Work out the finished part from the listing and answer in its coordinate system (mm). A direction names the side the tool comes from. Round coordinates to 2 decimals unless told otherwise and drop trailing zeros. Loops run counter-clockwise (first coordinate to the right, second up) from the corner with the lowest first, then second, coordinate; pieces in that order, holes last. Notation, with made-up numbers: (0, 10) - (27, 10) arc R19 ccw to (27, 42) - close; hole circle Ø10 at (21, 9.5). An arc over 180 degrees is marked (long way). Return JSON: item names as keys, results as strings.
from build123d import *

# Parameters (mm, degrees)
BOSS_EXTRUDE1_DEPTH      = 5
BOSS_EXTRUDE1_DEPTH_BACK = 5
SKETCH1_W                = 32.8
SKETCH1_H                = 137
CUT_EXTRUDE1_DEPTH       = 2.8
CUT_EXTRUDE1_DEPTH_BACK  = 2.8
SKETCH1_4_R              = 4.9
CUT_EXTRUDE3_DEPTH       = 2.8
CUT_EXTRUDE3_DEPTH_BACK  = 2.8
SKETCH1_8_W              = 2
SKETCH1_8_H              = 2
SKETCH1_8_W_2            = 9.8
BOSS_EXTRUDE2_START      = 2.6
SKETCH1_5_W              = 8.1
SKETCH1_5_H              = 8.6
SKETCH1_5_R              = 2.15
BOSS_EXTRUDE2_DEPTH      = 2.4
BOSS_EXTRUDE3_START      = -5
SKETCH1_6_W              = 8.1
SKETCH1_6_H              = 8.6
SKETCH1_6_R              = 2.15
BOSS_EXTRUDE3_DEPTH      = 2.4
FILLET1_R                = 5
CUT_EXTRUDE4_DEPTH       = 141.960419977
CUT_EXTRUDE4_DEPTH_BACK  = 141.960419977
SKETCH3_R                = 2.15


with BuildPart() as part:
    # Sketch1 → Boss-Extrude1 (new, two sides: drawn at the far end of the back side and taken through both)
    with BuildSketch(Plane(origin=(0, 0, 0), x_dir=(1, 0, 0), z_dir=(0, 1, 0)).offset(-BOSS_EXTRUDE1_DEPTH_BACK)):
        with Locations((16.4, -68.5)):
            Rectangle(SKETCH1_W, SKETCH1_H)
        with BuildLine():
            Line((9, -135), (9, -10.5))
            ThreePointArc((9, -10.5), (13.9, -5.6), (18.8, -10.5))
            Line((18.8, -10.5), (18.8, -135))
            Line((18.8, -135), (9, -135))
        make_face(mode=Mode.SUBTRACT)
    extrude(amount=BOSS_EXTRUDE1_DEPTH + BOSS_EXTRUDE1_DEPTH_BACK)

    # Sketch1<4> → Cut-Extrude1 (cut, two sides: drawn at the far end of the back side and taken through both)
    with BuildSketch(Plane(origin=(0, 0, 0), x_dir=(1, 0, 0), z_dir=(0, 1, 0)).offset(-CUT_EXTRUDE1_DEPTH_BACK)):
        with BuildLine():
            Line((7, -10.5), (7, -135))
            Line((7, -135), (9, -135))
            Line((9, -135), (9, -15.357983121))
            ThreePointArc((9, -15.357983121), (7.519561144, -13.126785107), (7, -10.5))
        make_face()
        with BuildLine():
            Line((18.8, -135), (20.8, -135))
            Line((20.8, -135), (20.8, -10.5))
            ThreePointArc((20.8, -10.5), (20.280438856, -13.126785107), (18.8, -15.357983121))
            Line((18.8, -15.357983121), (18.8, -135))
        make_face()
        with BuildLine():
            Line((9, -15.357983121), (9, -135))
            Line((9, -135), (18.8, -135))
            Line((18.8, -135), (18.8, -15.357983121))
            ThreePointArc((18.8, -15.357983121), (13.9, -17.4), (9, -15.357983121))
        make_face()
        with BuildLine():
            ThreePointArc((20.8, -10.5), (13.9, -3.6), (7, -10.5))
            ThreePointArc((7, -10.5), (7.519561144, -13.126785107), (9, -15.357983121))
            Line((9, -15.357983121), (9, -10.5))
            ThreePointArc((9, -10.5), (13.9, -5.6), (18.8, -10.5))
            Line((18.8, -10.5), (18.8, -15.357983121))
            ThreePointArc((18.8, -15.357983121), (20.280438856, -13.126785107), (20.8, -10.5))
        make_face()
        with BuildLine():
            Line((9, -10.5), (9, -15.357983121))
            ThreePointArc((9, -15.357983121), (13.9, -17.4), (18.8, -15.357983121))
            Line((18.8, -15.357983121), (18.8, -10.5))
            ThreePointArc((18.8, -10.5), (13.9, -15.4), (9, -10.5))
        make_face()
        with Locations((13.9, -10.5)):
            Circle(SKETCH1_4_R)
    extrude(amount=CUT_EXTRUDE1_DEPTH + CUT_EXTRUDE1_DEPTH_BACK, mode=Mode.SUBTRACT)

    # Sketch1<8> → Cut-Extrude3 (cut, two sides: drawn at the far end of the back side and taken through both)
    with BuildSketch(Plane(origin=(0, 0, 0), x_dir=(1, 0, 0), z_dir=(0, 1, 0)).offset(-CUT_EXTRUDE3_DEPTH_BACK)):
        with Locations((8, -136)):
            Rectangle(SKETCH1_8_W, SKETCH1_8_H)
        with Locations((19.8, -136)):
            Rectangle(SKETCH1_8_W, SKETCH1_8_H)
        with Locations((13.9, -136)):
            Rectangle(SKETCH1_8_W_2, SKETCH1_8_H)
    extrude(amount=CUT_EXTRUDE3_DEPTH + CUT_EXTRUDE3_DEPTH_BACK, mode=Mode.SUBTRACT)

    # Sketch1<5> → Boss-Extrude2 (add)
    with BuildSketch(Plane(origin=(0, 0, 0), x_dir=(1, 0, 0), z_dir=(0, 1, 0)).offset(BOSS_EXTRUDE2_START)):
        with Locations((20.25, 4.3)):
            Rectangle(SKETCH1_5_W, SKETCH1_5_H)
        with Locations(Location((20.25, 4.55, 0), (0, 0, 270))):
            Circle(SKETCH1_5_R, mode=Mode.SUBTRACT)
    extrude(amount=BOSS_EXTRUDE2_DEPTH)

    # Sketch1<6> → Boss-Extrude3 (add)
    with BuildSketch(Plane(origin=(0, 0, 0), x_dir=(1, 0, 0), z_dir=(0, 1, 0)).offset(BOSS_EXTRUDE3_START)):
        with Locations((20.25, 4.3)):
            Rectangle(SKETCH1_6_W, SKETCH1_6_H)
        with Locations(Location((20.25, 4.55, 0), (0, 0, 270))):
            Circle(SKETCH1_6_R, mode=Mode.SUBTRACT)
    extrude(amount=BOSS_EXTRUDE3_DEPTH)

    # Mirror1: part across plane


with BuildPart() as part_1:
    add(part.part)
    add(part.part.mirror(Plane(origin=(0, 0, 0), x_dir=(0, 0, 1), z_dir=(1, 0, 0))))

    # Fillet1
    fillet1_edges = [part_1.edges().sort_by_distance(p)[0] for p in [
        (-7, 0, 137),
        (7, 0, 137),
    ]]
    fillet(fillet1_edges, radius=FILLET1_R)

    # Sketch3 → Cut-Extrude4 (cut, two sides: drawn at the far end of the back side and taken through both)
    with BuildSketch(Plane(origin=(0, 0, 0), x_dir=(1, 0, 0), z_dir=(0, 1, 0)).offset(-CUT_EXTRUDE4_DEPTH_BACK)):
        with Locations(Location((0, -132, 0), (0, 0, 270))):
            Circle(SKETCH3_R)
        with Locations(Location((26.8, -132, 0), (0, 0, 270))):
            Circle(SKETCH3_R)
        with Locations(Location((-26.8, -132, 0), (0, 0, 270))):
            Circle(SKETCH3_R)
    extrude(amount=CUT_EXTRUDE4_DEPTH + CUT_EXTRUDE4_DEPTH_BACK, mode=Mode.SUBTRACT)


solid = part_1.part
1) Section B-B (x = -26.8) is taken. Give the vertices of the cut face in (y, z), and give its area (3 significant figures).
Verdict:
{"outline": "(-5, 0) - (5, 0) - (5, 129.85) - (-5, 129.85) - close; (-5, 134.15) - (5, 134.15) - (5, 137) - (-5, 137) - close", "area": "1,330 mm2"}
2) Section C-C (y = 0) is taken. Give the vertices of the cut face in (x, z), and give its area (3 significant figures).
Verdict:
{"outline": "(-32.8, 0) - (32.8, 0) - (32.8, 137) - (20.8, 137) - (20.8, 10.5) arc R6.9 cw to (7, 10.5) - (7, 132) arc R5 ccw to (2, 137) - (-2, 137) arc R5 ccw to (-7, 132) - (-7, 10.5) arc R6.9 cw to (-20.8, 10.5) - (-20.8, 137) - (-32.8, 137) - close; hole circle Ø4.3 at (-26.8, 132); hole circle Ø4.3 at (0, 132); hole circle Ø4.3 at (26.8, 132)", "area": "5,290 mm2"}
3) Section D-D (x = 11) is taken. Give the vertices of the cut face in (y, z), and give its area (3 significant figures).
Verdict:
{"outline": "(-5, 0) - (5, 0) - (5, 6.55) - (2.8, 6.55) - (2.8, 4.24) - (-2.8, 4.24) - (-2.8, 6.55) - (-5, 6.55) - close; (-5, 135) - (-2.8, 135) - (-2.8, 137) - (-5, 137) - close; (2.8, 135) - (5, 135) - (5, 137) - (2.8, 137) - close", "area": "61.4 mm2"}
4) Flat-ended cylindrical pins translate along their axes: pin 1 (0.7 mm diameter, centred on y = -3.5, z = -3, fed in from -X); pin 2 (0.7 mm diameter, centred on x = 12, y = 3.5, fed in from -Z); pin 3 (1.2 mm diameter, centred on y = 4, z = -4.5, fed in from +X). Find the tip coordinate at first contact, or state that the pin passes through.
Verdict:
{"pin 1": "stops at x = -24.3", "pin 2": "stops at z = 0", "pin 3": "stops at x = 24.3"}
5) A tool of negligible diameter and unlimited length cuts with its end or side. For faces 5 (the cylindrical face through (-13.8, 3.9, 5.6)), 6 (the flat face through (32.8, 0, 69)), 7 (the flat face through (0, -5, 63)), 8 (the cylindrical face through (5, 0, 136)), 9 (the flat face through (-18, 2.6, -3)), from which of +Z, -Z, +X, -X, +Y, -Y can it reach the whole face along a straight path? Write none if from no direction.
Verdict:
{"face 5": "+Y, -Y", "face 6": "+Z, -Z, +X, +Y, -Y", "face 7": "+Z, -Z, +X, -X, -Y", "face 8": "+Z", "face 9": "-Z, +X, -X"}
6) Section A-A (z = 90.5) is taken. Give the vertices of the cut face in (x, y).
Verdict:
{"outline": "(-32.8, -5) - (-18.8, -5) - (-18.8, -2.8) - (-20.8, -2.8) - (-20.8, 2.8) - (-18.8, 2.8) - (-18.8, 5) - (-32.8, 5) - close; (-9, -5) - (9, -5) - (9, -2.8) - (7, -2.8) - (7, 2.8) - (9, 2.8) - (9, 5) - (-9, 5) - (-9, 2.8) - (-7, 2.8) - (-7, -2.8) - (-9, -2.8) - close; (18.8, -5) - (32.8, -5) - (32.8, 5) - (18.8, 5) - (18.8, 2.8) - (20.8, 2.8) - (20.8, -2.8) - (18.8, -2.8) - close"}
7) Find the intervals of material crossed by L1, parallel to X at y = 3.25, z = 73.5; L2, parallel to X at y = -3, z = 132; L3, parallel to X at y = 1, z = 132, in increasing order.
Verdict:
{"L1": "x = -32.8 to -18.8, -9 to 9, 18.8 to 32.8", "L2": "x = -32.8 to -28.95, -24.65 to -18.8, -9 to -2.15, 2.15 to 9, 18.8 to 24.65, 28.95 to 32.8", "L3": "x = -32.8 to -28.95, -24.65 to -20.8, -7 to -2.15, 2.15 to 7, 20.8 to 24.65, 28.95 to 32.8"}
8) Determine the mould class of faces 1 (the cylindrical face through (13.8, 3.9, 5.6)), 2 (the cylindrical face through (18.34, -3.82, -3.56)), 3 (the flat face through (0, 5, 63)), 4 (the cylindrical face through (-5, 0, 136)) for opening direction Z: pulls with the +Z half, pulls with the -Z half, needs draft (parallel to the pull), parting line crosses it, or undercut.
Verdict:
{"face 1": "undercut", "face 2": "undercut", "face 3": "needs draft", "face 4": "pulls with the +Z half"}
